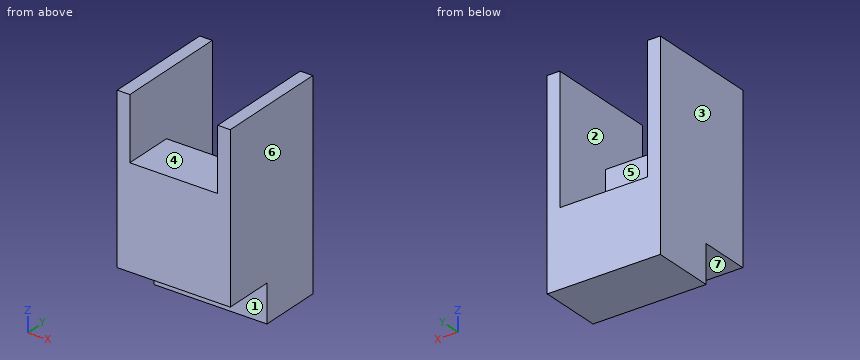
from build123d import *

# Parameters (mm, degrees)
F0_W     = 45
F0_H     = 45
F1_DEPTH = 80
F2_W     = 35
F2_H     = 20
F4_DEPTH = 25
F2_H_2   = 25
F5_DEPTH = 50
F3_W     = 45
F3_H     = 15
F6_DEPTH = 20


with BuildPart() as f1:
    # F0 (on Top) → F1 (new body)
    with BuildSketch(Plane.XY):
        Rectangle(F0_W, F0_H)
    extrude(amount=F1_DEPTH)

    # F2 (on face) → F4 (cut)
    with BuildSketch(Plane.XY.offset(80)):
        with Locations((0, -12.5)):
            Rectangle(F2_W, F2_H)
    extrude(amount=-F4_DEPTH, mode=Mode.SUBTRACT)

    # F2 (on face) → F5 (cut)
    with BuildSketch(Plane.XY.offset(80)):
        with Locations((0, 10)):
            Rectangle(F2_W, F2_H_2)
    extrude(amount=-F5_DEPTH, mode=Mode.SUBTRACT)

    # F3 (on face) → F6 (cut)
    with BuildSketch(Plane.XZ.offset(22.5)):
        with Locations((0, 7.5)):
            Rectangle(F3_W, F3_H)
    extrude(amount=-F6_DEPTH, mode=Mode.SUBTRACT)


solid = f1.part
Could you check a few things on this model? Use its own coordinates, in mm. Face numbers are marked on the shaded views. A direction names the side the tool comes from. Round coordinates to 2 decimals unless told otherwise and drop trailing zeros. Write each loop counter-clockwise with the first axis right and the second up, starting at its lowest first coordinate (ties: lowest second). Pieces come first, ordered by that corner, then holes. Notation, with made-up numbers: (79, 38.25) - (90, 38.25) arc R10 cw to (90, 48.25) - close; hole circle Ø5 at (53, -36.75). An arc over 180 degrees is marked (long way). Put each result on its own line as item: value. Start each with the question number.
(1) I want a section at C-C, the plane z = 39. Please give me the cut outline in (x, y).
(2) I need wall thicknesses on probe 1 along X at (y, z) = (-2, 61); probe 2 along Y at (x, z) = (20, 10.5); probe 3 along Z at (x, y) = (-1.5, -16). Which ranges of each line are inside material? Lowest first, please.
(3) I want a section at B-B, the plane y = 16. Please give me the cut outline in (x, z).
(4) For the marked faces 1, 2 and 3, which set-ups out of +Z, -Z, +X, -X, +Y, -Y let a thin tool reach every point of the face, with its end or its side?
(5) Thinking about a two-plate mould opening in X: for the marked faces 4, 5, 6 and 7, which applies, released by +X, released by -X, zero draft, split by the parting line, or undercut?
(6) Will these pins go through, and if not, where does the flat tip stop? pin 1 (8 mm diameter, centred on x = 7, y = -11.5, fed in from -Z); pin 2 (12 mm diameter, centred on x = -15.5, y = -6.5, fed in from -Z); pin 3 (6 mm diameter, centred on x = -4.5, y = -15.5, fed in from +Z); pin 4 (7.5 mm diameter, centred on x = 6, z = 42.5, fed in from +Y).
(7) I want a section at A-A, the plane z = 60.5. Please give me the cut outline in (x, y).
Here are the results:
1. outline: (-22.5, -22.5) - (22.5, -22.5) - (22.5, 22.5) - (17.5, 22.5) - (17.5, -2.5) - (-17.5, -2.5) - (-17.5, 22.5) - (-22.5, 22.5) - close
2. probe 1: x = -22.5 to -17.5, 17.5 to 22.5
2. probe 2: y = -2.5 to 22.5
2. probe 3: z = 15 to 55
3. outline: (-22.5, 0) - (22.5, 0) - (22.5, 80) - (17.5, 80) - (17.5, 30) - (-17.5, 30) - (-17.5, 80) - (-22.5, 80) - close
4. face 1: -Z, +X, -X, -Y
4. face 2: +Z, +Y
4. face 3: +Z, -Z, -X, +Y, -Y
5. face 4: undercut
5. face 5: undercut
5. face 6: released by +X
5. face 7: zero draft
6. pin 1: stops at z = 15
6. pin 2: stops at z = 0
6. pin 3: stops at z = 55
6. pin 4: stops at y = -2.5
7. outline: (-22.5, -22.5) - (-17.5, -22.5) - (-17.5, 22.5) - (-22.5, 22.5) - close; (17.5, -22.5) - (22.5, -22.5) - (22.5, 22.5) - (17.5, 22.5) - close
